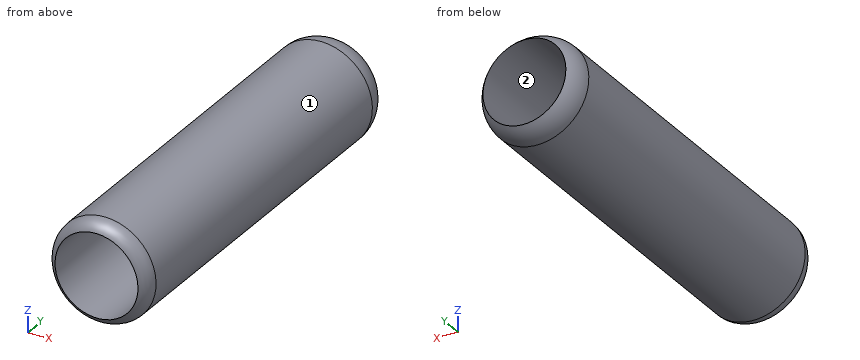
```python
from build123d import *

# Parameters (mm, degrees)
SKETCH3_R           = 15.5
SKETCH3_R_2         = 12.7
BOSS_EXTRUDE5_DEPTH = 120
FILLET5_R           = 10
FILLET6_R           = 5


with BuildPart() as part:
    # Sketch3 → Boss-Extrude5 (new body)
    with BuildSketch(Plane(origin=(0, 0, 0), x_dir=(1, 0, 0), z_dir=(0, 1, 0))):
        with Locations(Location((0, 0, 0), (0, 0, 270))):
            Circle(SKETCH3_R)
        with Locations(Location((0, 0, 0), (0, 0, 270))):
            Circle(SKETCH3_R_2, mode=Mode.SUBTRACT)
    extrude(amount=BOSS_EXTRUDE5_DEPTH)

    # Fillet5
    # the kernel refuses this fillet: 10 mm, written as the material it takes off along each edge
    with BuildSketch(Plane(origin=(0, 120, 0), x_dir=(0, 0, 1), z_dir=(-1, 0, 0))) as fillet5_piece_1:
        with BuildLine():
            CenterArc((5.5, -6.939740629), FILLET5_R, 0, 43.945519562)
            Line((12.7, 0), (12.844, 0.138794813))
            ThreePointArc((12.844, 0.138794813), (14.1, 0.2), (15.5, 0.2))
            Line((15.5, 0.2), (15.7, 0))
            Line((15.7, 0), (15.7, -6.939740629))
            Line((15.7, -6.939740629), (15.5, -6.939740629))
        make_face()
    revolve(axis=Axis((0, 120, 0), (0, 1, 0)), mode=Mode.SUBTRACT)

    # Fillet6
    # the kernel refuses this fillet: 5 mm, written as the material it takes off along each edge
    with BuildSketch(Plane(origin=(0, 0, 0), x_dir=(0, 0, 1), z_dir=(-1, 0, 0))) as fillet6_piece_1:
        with BuildLine():
            CenterArc((10.5, 4.489988864), FILLET6_R, 296.103881137, 63.896118863)
            Line((12.7, 0), (12.744, -0.089799777))
            ThreePointArc((12.744, -0.089799777), (14.1, -0.1), (15.5, -0.1))
            Line((15.5, -0.1), (15.6, 0))
            Line((15.6, 0), (15.6, 4.489988864))
            Line((15.6, 4.489988864), (15.5, 4.489988864))
        make_face()
    revolve(axis=Axis((0, 0, 0), (0, 1, 0)), mode=Mode.SUBTRACT)


solid = part.part
```
The model under review builds one solid part; all positions refer to its coordinate system, in mm. Face numbers are marked on the shaded views. Round coordinates to 2 decimals unless told otherwise and drop trailing zeros. Loops run counter-clockwise (first coordinate to the right, second up) from the corner with the lowest first, then second, coordinate; pieces in that order, holes last.
1) The part is to be moulded in two halves that separate along X. For the marked faces 1 and 2, say which applies: pulls with the +X half, pulls with the -X half, needs draft (parallel to the pull), parting line crosses it, or undercut.
Values follow:
face 1: parting line crosses it
face 2: undercut
2) Clearance check with flat-ended pins moving along their axes: P1, Ø10, axis at x = 11.5, y = 32.5, coming from the +Z side; P2, Ø8, axis at y = 99, z = 5, coming from the -X side; P3, Ø12, axis at x = 9.5, y = 33.5, coming from the -Z side. State where each tip first meets the part, or that it passes through.
Values follow:
P1: stops at z = 14.07
P2: stops at x = -15.47
P3: stops at z = -15.1
3) Consider section A-A on y = 28.5. State the section outline as (x, z) points, then the cut area to 3 significant figures.
Values follow:
outline: circle Ø31 at (0, 0); hole circle Ø25.4 at (0, 0)
area: 248 mm2
4) Wall thickness on line 1 along X through (y, z) = (92.5, 0); line 2 along Z through (x, y) = (-11, 32); line 3 along Z through (x, y) = (4, 93): over which ranges is each line inside the solid? List them lowest first.
Values follow:
line 1: x = -15.5 to -12.7, 12.7 to 15.5
line 2: z = -10.92 to -6.35, 6.35 to 10.92
line 3: z = -14.97 to -12.05, 12.05 to 14.97
